Work out the finished part from the listing and answer in its coordinate system (mm). Face numbers are marked on the shaded views. Give positions to 0.01 mm unless a question says otherwise; leave off trailing zeros. Loops run counter-clockwise (first coordinate to the right, second up) from the corner with the lowest first, then second, coordinate; pieces in that order, holes last. Notation, with made-up numbers: M 68,6 L 99,6 A17 cw 99,39 Z; hole C 8,80.5 d1. An arc over 180 degrees is marked long. Use a Markdown table: item, result.
```python
from build123d import *

# Parameters (mm, degrees)
SKETCH1_W                = 16.31
SKETCH1_H                = 4
BOSS_EXTRUDE3_DEPTH      = 5
CUT_EXTRUDE9_DEPTH       = 5
SKETCH4_R                = 1.5
CUT_EXTRUDE10_DEPTH      = 2.5
CUT_EXTRUDE10_DEPTH_BACK = 2.5


with BuildPart() as part:
    # Sketch1 → Boss-Extrude3 (new body)
    with BuildSketch(Plane.XY):
        Rectangle(SKETCH1_W, SKETCH1_H)
    extrude(amount=-BOSS_EXTRUDE3_DEPTH)

    # Sketch3 → Cut-Extrude9 (cut)
    with BuildSketch(Plane.XY):
        with BuildLine():
            Line((-3.355, -2), (3.355, -2))
            ThreePointArc((3.355, -2), (0, 1.355), (-3.355, -2))
        make_face()
    extrude(amount=-CUT_EXTRUDE9_DEPTH, mode=Mode.SUBTRACT)

    # Sketch4 → Cut-Extrude10 (cut, two sides)
    with BuildSketch(Plane(origin=(0, 0, 0), x_dir=(1, 0, 0), z_dir=(0, 1, 0))) as cut_extrude10_sk:
        with Locations((-5.755, 2.5)):
            Circle(SKETCH4_R)
        with Locations((5.755, 2.5)):
            Circle(SKETCH4_R)
    extrude(amount=CUT_EXTRUDE10_DEPTH, mode=Mode.SUBTRACT)
    extrude(cut_extrude10_sk.sketch, amount=-CUT_EXTRUDE10_DEPTH_BACK, mode=Mode.SUBTRACT)


solid = part.part
```
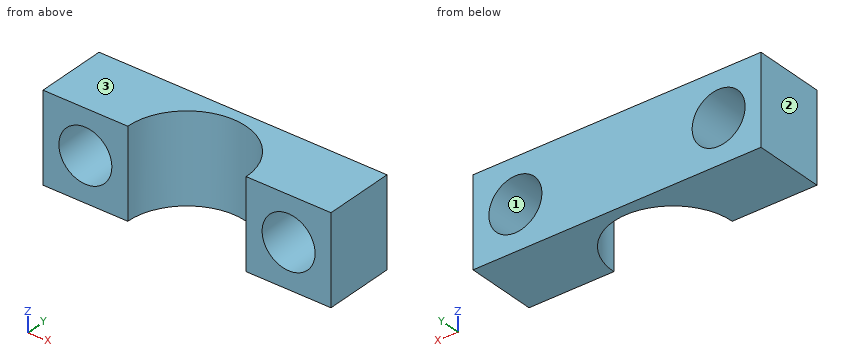
(1) A cutting plane is placed at A-A (y = -0.1). Write down the section's boundary in (x, z) (3 decimals), and give its area (3 significant figures).
Entries:
| item | result |
|---|---|
| outline | M -8.155,-5 L -2.765,-5 L -2.765,0 L -8.155,0 Z; M 2.765,-5 L 8.155,-5 L 8.155,0 L 2.765,0 Z; hole C -5.755,-2.5 d3; hole C 5.755,-2.5 d3 |
| area | 39.8 mm² |
(2) A cutting plane is placed at D-D (z = -4.55). Write down the section's boundary in (x, y) (3 decimals).
Entries:
| item | result |
|---|---|
| outline | M -8.155,-2 L -3.355,-2 A3.355 cw 3.355,-2 L 8.155,-2 L 8.155,2 L -8.155,2 Z |
(3) The mould has two halves that part along Z. Classify the marked faces 1, 2 and 3: released by +Z, released by -Z, zero draft, split by the parting line, or undercut.
Entries:
| item | result |
|---|---|
| face 1 | undercut |
| face 2 | zero draft |
| face 3 | released by +Z |
(4) Consider probe 1 along X at (y, z) = (-0.6, -2.5) (3 decimals); probe 2 along X at (y, z) = (-0.65, -2.5) (3 decimals); probe 3 along X at (y, z) = (0.3, -4.15) (3 decimals). Determine where each line is inside the solid, lowest interval first. Write a range as [from, to].
Entries:
| item | result |
|---|---|
| probe 1 | x = [-8.155, -7.255], [-4.255, -3.049], [3.049, 4.255], [7.255, 8.155] |
| probe 2 | x = [-8.155, -7.255], [-4.255, -3.071], [3.071, 4.255], [7.255, 8.155] |
| probe 3 | x = [-8.155, -2.443], [2.443, 8.155] |
(5) A cutting plane is placed at B-B (z = -2.5). Write down the section's boundary in (x, y) (3 decimals).
Entries:
| item | result |
|---|---|
| outline | M -8.155,-2 L -7.255,-2 L -7.255,2 L -8.155,2 Z; M -4.255,-2 L -3.355,-2 A3.355 cw 3.355,-2 L 4.255,-2 L 4.255,2 L -4.255,2 Z; M 7.255,-2 L 8.155,-2 L 8.155,2 L 7.255,2 Z |
(6) A cutting plane is placed at C-C (x = 4.5). Write down the section's boundary in (y, z).
Entries:
| item | result |
|---|---|
| outline | M -2,-5 L 2,-5 L 2,-3.32 L -2,-3.32 Z; M -2,-1.68 L 2,-1.68 L 2,0 L -2,0 Z |
